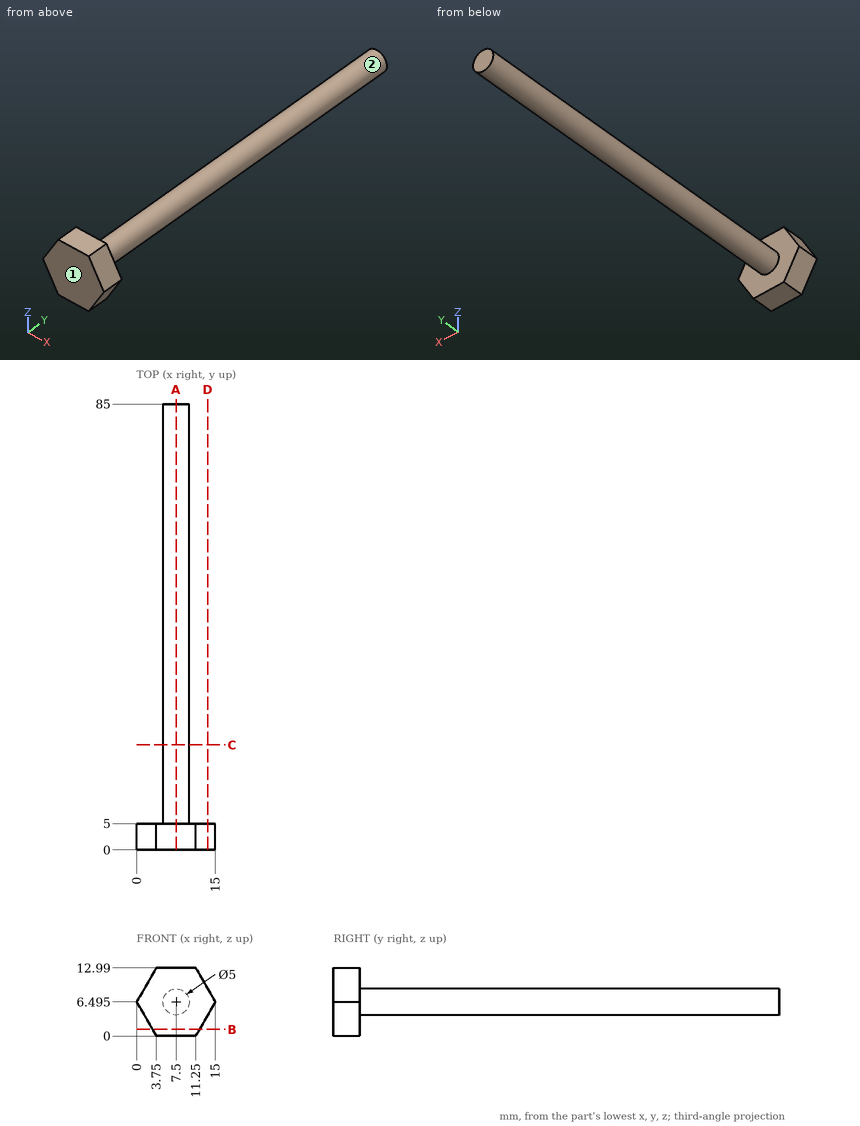
The figure shows three views and two pictorial views of one solid part (mm, origin at its lowest corner). Answer the questions. A direction names the side the tool comes from. Coordinates: 2 decimals unless noted, no trailing zeros. Order: outer loops, then holes, each group sorted by start corner. A loop starts at its lowest first (then second) coordinate and runs counter-clockwise, first axis right, second up. Notation, with made-up numbers: (-18.5, 0) - (-13.5, 0) arc R19 ccw to (-13.5, 8) - close; hole circle Ø5 at (27, 11.5). An arc over 180 degrees is marked (long way). Answer as a JSON object with one key per item and string values.
1. Find section A-A on x = 7.5. Determine the outline of the cut face in (y, z) (1 decimal).
Output values:
{"outline": "(0, 0) - (5, 0) - (5, 4) - (85, 4) - (85, 9) - (5, 9) - (5, 13) - (0, 13) - close"}
2. A tool of negligible diameter and unlimited length cuts with its end or side. For the marked faces 1 and 2, from which of +Z, -Z, +X, -X, +Y, -Y can it reach the whole face along a straight path? Write none if from no direction.
Output values:
{"face 1": "+Z, -Z, +X, -X, -Y", "face 2": "+Y"}
3. Each of these flat-tipped pins is pushed along its axis until it touches: P1, Ø5, axis at y = 61, z = 10, coming from the -X side; P2, Ø5, axis at x = 11, y = 14.5, coming from the -Z side; P3, Ø8, axis at x = 9.5, y = 44.5, coming from the -Z side (1 decimal). Where does it stop, or does it pass through?
Output values:
{"P1": "stops at x = 5.21", "P2": "stops at z = 4.2", "P3": "stops at z = 4"}
4. Consider line 1 (Y direction, x = 12, z = 10); line 2 (Z direction, x = 9.5, y = 39.5) (1 decimal); line 3 (X direction, y = 77.5, z = 4.25). Determine where each line is inside the solid, lowest interval first.
Output values:
{"line 1": "y = 0 to 5", "line 2": "z = 5 to 8", "line 3": "x = 6.4 to 8.6"}
5. Find section C-C on y = 20. Determine the outline of the cut face in (x, z) (1 decimal).
Output values:
{"outline": "circle Ø5 at (7.5, 6.5)"}
6. Find section D-D on x = 13.5. Determine the outline of the cut face in (y, z).
Output values:
{"outline": "(0, 3.9) - (5, 3.9) - (5, 9.09) - (0, 9.09) - close"}
7. Find section B-B on z = 1.25. Determine the outline of the cut face in (x, y), plus the area to 3 significant figures.
Output values:
{"outline": "(3.03, 0) - (11.97, 0) - (11.97, 5) - (3.03, 5) - close", "area": "44.7 mm²"}
